Work out the finished part from the listing and answer in its coordinate system (mm). Face numbers are marked on the shaded views. Give positions to 0.01 mm unless a question says otherwise; leave off trailing zeros. Write each loop counter-clockwise with the first axis right and the second up, starting at its lowest first coordinate (ties: lowest second). Pieces come first, ordered by that corner, then holes.
1) Straight lines are drawn through the part: probe 1 along Z at (x, y) = (-12.5, 25); probe 2 along Y at (x, z) = (0, 1.85); probe 3 along X at (y, z) = (4, 0.55). For each, find the intervals that lie inside material, in ascending order.
2) Find section A-A (y = 0). Determine the outline of the cut face in (x, z), plus the area to 3 significant figures.
3) Given pin 1 Ø7 at (x, y) = (0, 0) entering from -Z; pin 2 Ø2.5 at (x, y) = (0, -7.3) entering from -Z; pin 3 Ø3 at (y, z) = (12, 1) entering from -X; pin 4 Ø3 at (y, z) = (3, -1.5) entering from +X, each flat-ended and moving along its own axis, determine where each tip first touches the part or whether it passes through.
4) Determine the mould class of the marked faces 1, 2 and 3 for opening direction X: pulls with the +X half, pulls with the -X half, needs draft (parallel to the pull), parting line crosses it, or undercut.
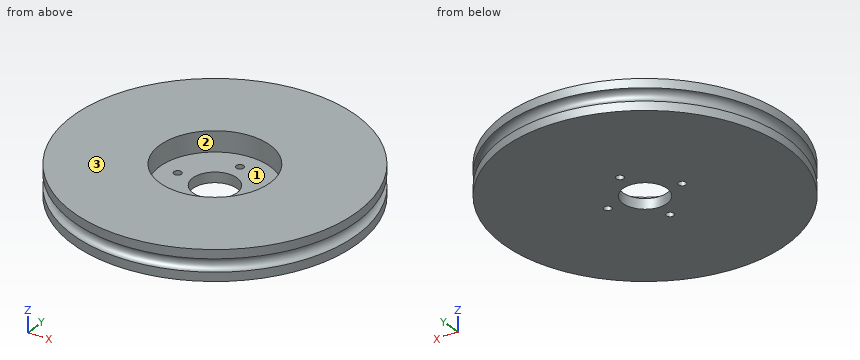
```python
from build123d import *

# Parameters (mm, degrees)
CYLINDER003_R     = 0.75
CYLINDER003_DEPTH = 10
ARRAY_COUNT       = 4
CYLINDER002_R     = 4.35
CYLINDER002_DEPTH = 10
CYLINDER001_R     = 10.9
CYLINDER001_DEPTH = 10
TORUS_R           = 1.25
CYLINDER_R        = 28
CYLINDER_DEPTH    = 6


with BuildPart() as array:
    # Cylinder003 → Cylinder003 (new body)
    with BuildSketch(Plane(origin=(7.3, 0, -5), x_dir=(1, 0, 0), z_dir=(0, 0, 1))):
        Circle(CYLINDER003_R)
    extrude(amount=CYLINDER003_DEPTH)

    # Array: Array ×4 about axis
    array_axis = Axis((0, 0, 0), (0, 0, 1))


with BuildPart() as array_1:
    add(array.part)
    for i in range(1, ARRAY_COUNT):
        add(array.part.rotate(array_axis, i * 360 / ARRAY_COUNT))


with BuildPart() as hueco_eje:
    # Cylinder002 → Cylinder002 (new body)
    with BuildSketch(Plane.XY.offset(-10)):
        Circle(CYLINDER002_R)
    extrude(amount=CYLINDER002_DEPTH)


with BuildPart() as cylinder:
    # Cylinder001 → Cylinder001 (new body)
    with BuildSketch(Plane.XY.offset(-1)):
        Circle(CYLINDER001_R)
    extrude(amount=CYLINDER001_DEPTH)


with BuildPart() as obj1:
    # Torus → Torus (revolve)
    with BuildSketch(Plane.XZ):
        with Locations((28, 0)):
            Circle(TORUS_R)
    revolve(axis=Axis((0, 0, 0), (0, 0, 1)))


with BuildPart() as cut003:
    # Cylinder → Cylinder (new body)
    with BuildSketch(Plane.XY.offset(-3)):
        Circle(CYLINDER_R)
    extrude(amount=CYLINDER_DEPTH)

    # Cut: cut obj1
    add(obj1.part, mode=Mode.SUBTRACT)

    # Cut001: cut Cylinder
    add(cylinder.part, mode=Mode.SUBTRACT)

    # Cut002: cut hueco_eje
    add(hueco_eje.part, mode=Mode.SUBTRACT)

    # Cut003: cut Array
    add(array_1.part, mode=Mode.SUBTRACT)


solid = cut003.part
```
Results:
1. probe 1: z = -3 to -1.25, 1.25 to 3
1. probe 2: y = -28 to -10.9, 10.9 to 28
1. probe 3: x = -26.58 to -10.14, 10.14 to 26.58
2. outline: (-28, -3) - (-8.05, -3) - (-8.05, -1) - (-10.9, -1) - (-10.9, 3) - (-28, 3) - (-28, 1.25) arc R1.25 cw to (-28, -1.25) - close; (-6.55, -3) - (-4.35, -3) - (-4.35, -1) - (-6.55, -1) - close; (4.35, -3) - (6.55, -3) - (6.55, -1) - (4.35, -1) - close; (8.05, -3) - (28, -3) - (28, -1.25) arc R1.25 cw to (28, 1.25) - (28, 3) - (10.9, 3) - (10.9, -1) - (8.05, -1) - close
2. area: 220 mm2
3. pin 1: passes through
3. pin 2: stops at z = -3
3. pin 3: stops at x = -25.95
3. pin 4: stops at x = 27.96
4. face 1: undercut
4. face 2: undercut
4. face 3: needs draft
